Check sheet for the modelled part. Datum: model origin and axes. Units: mm. Round coordinates to 2 decimals unless told otherwise and drop trailing zeros. Loops run counter-clockwise (first coordinate to the right, second up) from the corner with the lowest first, then second, coordinate; pieces in that order, holes last. Notation, with made-up numbers: M 9.5,32 L 13.5,32 A8 ccw 13.5,47 Z; hole C -23.5,-38.75 d5. An arc over 180 degrees is marked long. One line per question, with ' | ' between items. Start each with the question number.
(1) Go/stop test with a flat-tipped pin: P1, Ø1.8, axis at x = 4.95, y = -4.95, coming from the -Z side. Record where the tip stops, or that it passes through.
(2) Section check D-D (z = 0.7). Count the separate pieces of the cut face and the enclosed holes in it, and give its area (3 significant figures).
(3) Section check C-C (x = 0). Record the boundary of the cut face in (y, z).
(4) Draft check along X on faces 1 (the face through (17.699, 17.715, 0.507)), 2 (the face through (-17.715, -17.699, 0.507)), 3 (the face through (-5.687, -4.274, 0.493)). Enter one of: +X half, -X half, draft (parallel to the pull), parting line (faces both ways), or undercut.
(5) Thickness scan on probe 1 along Y at (x, z) = (0, 0.7); probe 2 along X at (y, z) = (5.5, 0.9). Record the ranges inside material, lowest first. Write a range as [from, to].
(6) Section check A-A (y = -15). Record the boundary of the cut face in (x, z), and give its area (3 significant figures).
```python
from build123d import *

# Parameters (mm, degrees)
F0_W     = 36
F0_H     = 36
F0_R     = 1
F0_R_2   = 5.25
F1_DEPTH = 1
F2_R     = 1


with BuildPart() as f1:
    # F0 (on Top) → F1 (new body)
    with BuildSketch(Plane.XY):
        Rectangle(F0_W, F0_H)
        with Locations((-15, -15)):
            Circle(F0_R, mode=Mode.SUBTRACT)
        with Locations((-4.949747, -4.949747)):
            Circle(F0_R, mode=Mode.SUBTRACT)
        with Locations((15, -15)):
            Circle(F0_R, mode=Mode.SUBTRACT)
        with Locations((0, -7)):
            Circle(F0_R, mode=Mode.SUBTRACT)
        with Locations((4.949747, -4.949747)):
            Circle(F0_R, mode=Mode.SUBTRACT)
        with Locations((-7, 0)):
            Circle(F0_R, mode=Mode.SUBTRACT)
        with Locations((-4.949747, 4.949747)):
            Circle(F0_R, mode=Mode.SUBTRACT)
        with Locations((-15, 15)):
            Circle(F0_R, mode=Mode.SUBTRACT)
        Circle(F0_R_2, mode=Mode.SUBTRACT)
        with Locations((7, 0)):
            Circle(F0_R, mode=Mode.SUBTRACT)
        with Locations((0, 7)):
            Circle(F0_R, mode=Mode.SUBTRACT)
        with Locations((4.949747, 4.949747)):
            Circle(F0_R, mode=Mode.SUBTRACT)
        with Locations((15, 15)):
            Circle(F0_R, mode=Mode.SUBTRACT)
    extrude(amount=F1_DEPTH)

    # F2
    f2_edges = [f1.edges().sort_by_distance(p)[0] for p in [
        (-18, 18, 0.5),
        (18, 18, 0.5),
        (-18, -18, 0.5),
        (18, -18, 0.5),
    ]]
    fillet(f2_edges, radius=F2_R)


solid = f1.part
```
The answers:
1) P1: through
2) separate pieces: 1 | enclosed holes: 13 | area: 1,170 mm²
3) outline: M -18,0 L -8,0 L -8,1 L -18,1 Z; M -6,0 L -5.25,0 L -5.25,1 L -6,1 Z; M 5.25,0 L 6,0 L 6,1 L 5.25,1 Z; M 8,0 L 18,0 L 18,1 L 8,1 Z
4) face 1: +X half | face 2: -X half | face 3: undercut
5) probe 1: [-18, -8], [-6, -5.25], [5.25, 6], [8, 18] | probe 2: [-18, -5.78], [-4.11, 4.11], [5.78, 18]
6) outline: M -18,0 L -16,0 L -16,1 L -18,1 Z; M -14,0 L 14,0 L 14,1 L -14,1 Z; M 16,0 L 18,0 L 18,1 L 16,1 Z | area: 32.0 mm²
